CAD build for the part. Positions are in the model's coordinates, mm. A direction names the side the tool comes from. Coordinates: 2 decimals unless noted, no trailing zeros. Loops run counter-clockwise (first coordinate to the right, second up) from the corner with the lowest first, then second, coordinate; pieces in that order, holes last. Notation, with made-up numbers: (0.25, -13.75) -> (17.25, -13.75) arc R8 cw to (17.25, -2.75) -> close; hole circle Ø8 at (64, 17). An arc over 180 degrees is marked (long way). Return JSON: item names as keys, results as strings. Group by question number.
(1) Saw through at C-C on x = 0.5. Write the cut outline in (y, z), then the cut area to 4 significant figures.
(2) Saw through at D-D on y = 12. Write the cut outline in (x, z), then the cut area to 3 significant figures.
(3) Mould opens along Y. For faces 1 (the face through (0, 25, 0)), 2 (the face through (25, 0, 6)), 3 (the face through (-23.73, -0.54, -2.44)), 4 (the face through (0, 20, 0)) say: pulls with the +Y half, pulls with the -Y half, needs draft (parallel to the pull), parting line crosses it, or undercut.
(4) Saw through at B-B on z = 0. Write the cut outline in (x, y).
(5) Probe L1, parallel to Y at x = 23, z = 0; L2, parallel to X at y = -18.5, z = 17. List the from-to ranges inside material, lowest first.
(6) Flat gauge pin, fed straight in: pin 1 Ø6 at (x, z) = (-2.5, -9.5) entering from -Y. Where does the tip first touch, or does it go through?
(7) Tool access for faces 5 (the face through (-2.5, 0, 24)), 6 (the face through (23.73, -0.54, -2.44)), 7 (the face through (22.5, -3, 0)): list every direction of +Z, -Z, +X, -X, +Y, -Y with a clear straight run to the whole face (end or side of a thin tool).
(8) Saw through at A-A on y = 0. Write the cut outline in (x, z), then the cut area to 4 significant figures.
```python
from build123d import *

# Parameters (mm, degrees)
F0_W          = 50
F0_H          = 50
F1_DEPTH      = 25
F1_DEPTH_BACK = 25
F2_W          = 45
F2_H          = 45
F3_DEPTH      = 45
F4_W          = 5
F4_H          = 5
F5_DEPTH      = 5
F6_R          = 2.5
F7_DEPTH      = 50
F7_DEPTH_BACK = 25


with BuildPart() as f1:
    # F0 (on Top) → F1 (new body, two sides)
    with BuildSketch(Plane.XY) as f1_sk:
        Rectangle(F0_W, F0_H)
    extrude(amount=F1_DEPTH)
    extrude(f1_sk.sketch, amount=-F1_DEPTH_BACK)

    # F2 (on face) → F3 (cut)
    with BuildSketch(Plane.XZ.offset(25)):
        Rectangle(F2_W, F2_H)
    extrude(amount=-F3_DEPTH, mode=Mode.SUBTRACT)

    # F4 (on face) → F5 (cut)
    with BuildSketch(Plane.XY.offset(25)):
        Rectangle(F4_W, F4_H)
    extrude(amount=-F5_DEPTH, mode=Mode.SUBTRACT)

    # F6 (on Right) → F7 (cut, two sides)
    with BuildSketch(Plane.YZ) as f7_sk:
        Circle(F6_R)
    extrude(amount=-F7_DEPTH, mode=Mode.SUBTRACT)
    extrude(f7_sk.sketch, amount=F7_DEPTH_BACK, mode=Mode.SUBTRACT)


solid = f1.part
```
Geometry results:
{
 "1": {"outline": "(-25, -25) -> (25, -25) -> (25, 25) -> (2.5, 25) -> (2.5, 22.5) -> (20, 22.5) -> (20, -22.5) -> (-25, -22.5) -> close; (-25, 22.5) -> (-2.5, 22.5) -> (-2.5, 25) -> (-25, 25) -> close", "area": "462.5 mm²"},
 "2": {"outline": "(-25, -25) -> (25, -25) -> (25, 25) -> (-25, 25) -> close; hole (-22.5, -22.5) -> (22.5, -22.5) -> (22.5, 22.5) -> (-22.5, 22.5) -> close", "area": "475 mm²"},
 "3": {"face 1": "pulls with the +Y half", "face 2": "needs draft", "face 3": "undercut", "face 4": "pulls with the -Y half"},
 "4": {"outline": "(-25, -25) -> (-22.5, -25) -> (-22.5, -2.5) -> (-25, -2.5) -> close; (-25, 2.5) -> (-22.5, 2.5) -> (-22.5, 20) -> (22.5, 20) -> (22.5, 2.5) -> (25, 2.5) -> (25, 25) -> (-25, 25) -> close; (22.5, -25) -> (25, -25) -> (25, -2.5) -> (22.5, -2.5) -> close"},
 "5": {"L1": "-25 to -2.5, 2.5 to 25", "L2": "-25 to -22.5, 22.5 to 25"},
 "6": {"pin 1": "y = 20"},
 "7": {"face 5": "+Z", "face 6": "+X, -X", "face 7": "-Y"},
 "8": {"outline": "(-25, -25) -> (25, -25) -> (25, -2.5) -> (22.5, -2.5) -> (22.5, -22.5) -> (-22.5, -22.5) -> (-22.5, -2.5) -> (-25, -2.5) -> close; (-25, 2.5) -> (-22.5, 2.5) -> (-22.5, 22.5) -> (-2.5, 22.5) -> (-2.5, 25) -> (-25, 25) -> close; (2.5, 22.5) -> (22.5, 22.5) -> (22.5, 2.5) -> (25, 2.5) -> (25, 25) -> (2.5, 25) -> close", "area": "437.5 mm²"}
}
